from build123d import *

# Parameters (mm, degrees)
F0_W     = 38.1
F0_H     = 38.1
F0_W_2   = 33.528
F0_H_2   = 33.528
F1_DEPTH = 812.8
F3_DEPTH = 50.8


with BuildPart() as f1:
    # F0 (on Front) → F1 (new body)
    with BuildSketch(Plane.XZ):
        with Locations((-19.05, -19.05)):
            Rectangle(F0_W, F0_H)
        with Locations((-19.05, -19.05)):
            Rectangle(F0_W_2, F0_H_2, mode=Mode.SUBTRACT)
    extrude(amount=F1_DEPTH)

    # F2 (on face) → F3 (cut)
    with BuildSketch(Plane.XY):
        Polygon((0, -774.7), (-38.1, -812.8), (0, -812.8), align=None)
        Polygon((0, 0), (-38.1, 0), (0, -38.1), align=None)
    extrude(amount=-F3_DEPTH, mode=Mode.SUBTRACT)


solid = f1.part
Here's how the part is built. I have some questions about the finished solid (model axes, mm). A direction names the side the tool comes from. Give positions to 0.01 mm unless a question says otherwise; leave off trailing zeros. Loops run counter-clockwise (first coordinate to the right, second up) from the corner with the lowest first, then second, coordinate; pieces in that order, holes last. Notation, with made-up numbers: (38, -29.75) -> (87, -29.75) arc R13 ccw to (87, -18.75) -> close; hole circle Ø5 at (40, 45.25). An arc over 180 degrees is marked (long way). Answer as a JSON object with one key per item and string values. Group by question number.
Item 1: Thinking about a two-plate mould opening in Z: for faces 3 (the flat face through (-19, -401, -38.1)), 4 (the flat face through (-19, -401, 0)), 5 (the flat face through (-38.1, -401, -19)), 6 (the flat face through (-19, -401, -35.814)), which applies, pulls with the +Z half, pulls with the -Z half, needs draft (parallel to the pull), parting line crosses it, or undercut?
Item 2: Imagine slicing it at A-A on x = -30. Write out the boundary of the cut face in (y, z), then the cut area to 3 significant figures.
Item 3: Imagine slicing it at C-C on z = -13.5. Write out the boundary of the cut face in (x, y).
Item 4: Imagine slicing it at B-B on y = -563.5. Write out the boundary of the cut face in (x, z), then the cut area to 3 significant figures.
Item 5: On a 3-axis mill with a long thin cutter (end or side, diameter ignored), from which of +Z, -Z, +X, -X, +Y, -Y can I reach the whole of each face in a straight line? I mean faces 1 (the flat face through (-2.286, -401, -19)), 2 (the flat face through (0, -401, -19)). Say none if no direction works.
Item 6: I need wall thicknesses on L1, parallel to X at y = -420, z = -23.5; L2, parallel to Y at x = -1.5, z = -15.5. Which ranges of each line are inside material? Lowest first, please.
Item 7: Will this pin go through, and if not, where does the flat tip stop? pin 1 (12 mm diameter, centred on x = -14.5, z = -4.5, fed in from -Y).
Answer list:
{
 "1": {"face 3": "pulls with the -Z half", "face 4": "pulls with the +Z half", "face 5": "needs draft", "face 6": "undercut"},
 "2": {"outline": "(-804.7, -38.1) -> (-8.1, -38.1) -> (-8.1, -35.81) -> (-804.7, -35.81) -> close; (-804.7, -2.29) -> (-8.1, -2.29) -> (-8.1, 0) -> (-804.7, 0) -> close", "area": "3,640 mm2"},
 "3": {"outline": "(-38.1, -812.8) -> (-35.81, -810.51) -> (-35.81, -2.29) -> (-38.1, 0) -> close; (-2.29, -776.99) -> (0, -774.7) -> (0, -38.1) -> (-2.29, -35.81) -> close"},
 "4": {"outline": "(-38.1, -38.1) -> (0, -38.1) -> (0, 0) -> (-38.1, 0) -> close; hole (-35.81, -35.81) -> (-2.29, -35.81) -> (-2.29, -2.29) -> (-35.81, -2.29) -> close", "area": "327 mm2"},
 "5": {"face 1": "+Y, -Y", "face 2": "+Z, -Z, +X, +Y, -Y"},
 "6": {"L1": "x = -38.1 to -35.81, -2.29 to 0", "L2": "y = -776.2 to -36.6"},
 "7": {"pin 1": "stops at y = -794.78"}
}
